```python
from build123d import *

# Parameters (mm, degrees)
SKETCH_1_R          = 15.345
EXTRUDE_1_DEPTH     = 13.5
SKETCH_2_R          = 17.5
EXTRUDE_2_DEPTH     = 2
SKETCH_4_R          = 11
EXTRUDE_3_DEPTH     = 13
SKETCH_3_R          = 3
CUT_EXTRUDE_1_DEPTH = 51.482670294


with BuildPart() as part:
    # 草图1 → 凸台-拉伸1 (new, symmetric)
    with BuildSketch(Plane(origin=(0, 0, 0), x_dir=(1, 0, 0), z_dir=(0, 1, 0))):
        with Locations(Location((0, 0, 0), (0, 0, 270))):
            Circle(SKETCH_1_R)
    extrude(amount=EXTRUDE_1_DEPTH, both=True)

    # 草图2 → 凸台-拉伸2 (add)
    with BuildSketch(Plane(origin=(0, 13.5, 0), x_dir=(1, 0, 0), z_dir=(0, 1, 0))):
        with Locations(Location((0, 0, 0), (0, 0, 270))):
            Circle(SKETCH_2_R)
    extrude_2 = extrude(amount=EXTRUDE_2_DEPTH)

    # 镜向1: 凸台-拉伸2 across plane
    add(extrude_2.mirror(Plane.ZX))

    # 草图4 → 凸台-拉伸3 (add)
    with BuildSketch(Plane(origin=(0, 15.5, 0), x_dir=(1, 0, 0), z_dir=(0, 1, 0))):
        with Locations(Location((0.058014503, -0.029170846, 0), (0, 0, 90))):
            Circle(SKETCH_4_R)
    extrude(amount=EXTRUDE_3_DEPTH)

    # 草图3 → 切除-拉伸1 (cut, through all)
    with BuildSketch(Plane(origin=(0, -15.5, 0), x_dir=(1, 0, 0), z_dir=(0, 1, 0))):
        with Locations(Location((0, 0, 0), (0, 0, 270))):
            Circle(SKETCH_3_R)
    extrude(amount=CUT_EXTRUDE_1_DEPTH, mode=Mode.SUBTRACT)


solid = part.part
```
For this review, take the finished solid that the model builds, in its own axes (mm). A direction names the side the tool comes from. Round coordinates to 2 decimals unless told otherwise and drop trailing zeros. Write each loop counter-clockwise with the first axis right and the second up, starting at its lowest first coordinate (ties: lowest second). Pieces come first, ordered by that corner, then holes. Notation, with made-up numbers: (23, 38.5) - (34, 38.5) arc R17 ccw to (34, 43.5) - close; hole circle Ø9 at (-28, 28.5). An arc over 180 degrees is marked (long way). Put each result on its own line as item: value.
Q1. We need section C-C (y = 1.5). Give the boundary of the cut face in (x, z) (3 decimals), and give its area (3 significant figures).
Solved:
outline: circle Ø30.69 at (0, 0); hole circle Ø6 at (0, 0)
area: 711 mm2
Q2. We need section D-D (z = 13.5). Give the boundary of the cut face in (x, y).
Solved:
outline: (-11.14, -15.5) - (11.14, -15.5) - (11.14, -13.5) - (7.3, -13.5) - (7.3, 13.5) - (11.14, 13.5) - (11.14, 15.5) - (-11.14, 15.5) - (-11.14, 13.5) - (-7.3, 13.5) - (-7.3, -13.5) - (-11.14, -13.5) - close
Q3. Mouldability with a two-part tool opening along X and no side actions: class faces 1 (the face through (-15.5, -13.5, -0.1)), 2 (the face through (-10.648, -14.486, -13.887)), 3 (the face through (0.9, 6.19, 2.86)) as released by +X, released by -X, zero draft, split by the parting line, or undercut.
Solved:
face 1: zero draft
face 2: split by the parting line
face 3: undercut
Q4. We need section A-A (z = -1.5). Give the boundary of the cut face in (x, y).
Solved:
outline: (-17.44, -15.5) - (-2.6, -15.5) - (-2.6, 28.5) - (-10.84, 28.5) - (-10.84, 15.5) - (-17.44, 15.5) - (-17.44, 13.5) - (-15.27, 13.5) - (-15.27, -13.5) - (-17.44, -13.5) - close; (2.6, -15.5) - (17.44, -15.5) - (17.44, -13.5) - (15.27, -13.5) - (15.27, 13.5) - (17.44, 13.5) - (17.44, 15.5) - (10.95, 15.5) - (10.95, 28.5) - (2.6, 28.5) - close
Q5. Wall thickness on probe 1 along X at (y, z) = (14, 0); probe 2 along Z at (x, y) = (0, 17); probe 3 along Y at (x, z) = (0, 11.5): over which ranges is each line inside the solid? List them lowest first.
Solved:
probe 1: x = -17.5 to -3, 3 to 17.5
probe 2: z = -10.97 to -3, 3 to 11.03
probe 3: y = -15.5 to 15.5
Q6. Insertion check: pin 1 Ø2 at (y, z) = (-1.5, 2) entering from -X; pin 2 Ø3 at (y, z) = (-7.5, -1) entering from +X (3 decimals); pin 3 Ø3 at (x, y) = (-3.5, 21.5) entering from -Z. Each pin has a flat end and moves straight along its axis. Give the tip position at first contact, or say it passes through.
Solved:
pin 1: stops at x = -15.31
pin 2: stops at x = 15.345
pin 3: stops at z = -10.78
Q7. Machinability: for faces 4 (the face through (-4, -15.5, 0)), 5 (the face through (10.37, 0.19, -11.31)), 6 (the face through (-0.43, 21.91, 11.02)), which of the approach directions +Z, -Z, +X, -X, +Y, -Y give a long, thin tool a straight path to every point of the face, cutting with its end or side? Answer none if there is none.
Solved:
face 4: +Z, -Z, +X, -X, -Y
face 5: none
face 6: +Y
Q8. We need section B-B (x = 7). Give the boundary of the cut face in (y, z).
Solved:
outline: (-15.5, -16.04) - (-13.5, -16.04) - (-13.5, -13.66) - (13.5, -13.66) - (13.5, -16.04) - (15.5, -16.04) - (15.5, -8.5) - (28.5, -8.5) - (28.5, 8.56) - (15.5, 8.56) - (15.5, 16.04) - (13.5, 16.04) - (13.5, 13.66) - (-13.5, 13.66) - (-13.5, 16.04) - (-15.5, 16.04) - close
